from build123d import *

# Parameters (mm, degrees)
SKETCH1_W           = 130
SKETCH1_H           = 100
BOSS_EXTRUDE1_DEPTH = 51
SKETCH2_W           = 120
SKETCH2_H           = 90
CUT_EXTRUDE1_DEPTH  = 46
FILLET2_R           = 5
FILLET4_R           = 5
SKETCH6_W           = 5
SKETCH6_H           = 5
BOSS_EXTRUDE2_DEPTH = 20
BOSS_EXTRUDE3_DEPTH = 3


# Some blends are built 0.0001 mm under size
with BuildPart() as part:
    # Sketch1 → Boss-Extrude1 (new body)
    with BuildSketch(Plane(origin=(0, 0, 0), x_dir=(1, 0, 0), z_dir=(0, 1, 0))):
        Rectangle(SKETCH1_W, SKETCH1_H)
    extrude(amount=BOSS_EXTRUDE1_DEPTH)

    # Sketch2 → Cut-Extrude1 (cut)
    with BuildSketch(Plane(origin=(0, 51, 0), x_dir=(1, 0, 0), z_dir=(0, 1, 0))):
        Rectangle(SKETCH2_W, SKETCH2_H)
    extrude(amount=-CUT_EXTRUDE1_DEPTH, mode=Mode.SUBTRACT)

    # Fillet2
    fillet2_edges = [part.edges().sort_by_distance(p)[0] for p in [
        (-65, 51, 0),
        (0, 51, 50),
        (65, 51, 0),
        (0, 51, -50),
    ]]
    fillet(fillet2_edges, radius=FILLET2_R - 0.0001)  # a hair under: the kernel refuses the full size

    # Fillet4
    # the kernel refuses this fillet: 5 mm, written as the material it takes off along each edge
    with BuildSketch(Plane(origin=(60, 51, 45), x_dir=(0, 0, 1), z_dir=(-1, 0, 0))) as fillet4_piece_1:
        with BuildLine():
            CenterArc((0.0001, -4.9999), 4.9999, 0, 90)
            Line((5, -4.9999), (5, 0))
            Line((5, 0), (0.0001, 0))
        make_face()
    revolve(axis=Axis((60, 51, 45), (0, 1, 0)), revolution_arc=90, mode=Mode.SUBTRACT)
    with BuildSketch(Plane(origin=(-60, 51, 45), x_dir=(-1, 0, 0), z_dir=(0, 0, -1))) as fillet4_piece_2:
        with BuildLine():
            CenterArc((0.0001, -4.9999), 4.9999, 0, 90)
            Line((5, -4.9999), (5, 0))
            Line((5, 0), (0.0001, 0))
        make_face()
    revolve(axis=Axis((-60, 51, 45), (0, 1, 0)), revolution_arc=90, mode=Mode.SUBTRACT)
    with BuildSketch(Plane(origin=(60, 51, -45), x_dir=(1, 0, 0), z_dir=(0, 0, 1))) as fillet4_piece_3:
        with BuildLine():
            CenterArc((0.0001, -4.9999), 4.9999, 0, 90)
            Line((5, -4.9999), (5, 0))
            Line((5, 0), (0.0001, 0))
        make_face()
    revolve(axis=Axis((60, 51, -45), (0, 1, 0)), revolution_arc=90, mode=Mode.SUBTRACT)
    with BuildSketch(Plane(origin=(-60, 51, -45), x_dir=(0, 0, -1), z_dir=(1, 0, 0))) as fillet4_piece_4:
        with BuildLine():
            CenterArc((0.0001, -4.9999), 4.9999, 0, 90)
            Line((5, -4.9999), (5, 0))
            Line((5, 0), (0.0001, 0))
        make_face()
    revolve(axis=Axis((-60, 51, -45), (0, 1, 0)), revolution_arc=90, mode=Mode.SUBTRACT)
    with BuildSketch(Plane(origin=(-65, -12.5, -50), x_dir=(1, 0, 0), z_dir=(0, 1, 0)), Plane(origin=(-65, -12.5, 50), x_dir=(0, 0, -1), z_dir=(0, 1, 0))) as fillet4_piece_5:
        with BuildLine():
            CenterArc((FILLET4_R, -FILLET4_R), FILLET4_R, 90, 90)
            Line((0, -FILLET4_R), (0, 0))
            Line((0, 0), (FILLET4_R, 0))
        make_face()
    extrude(amount=63.5, mode=Mode.SUBTRACT)
    with BuildSketch(Plane(origin=(65, -12.5, -50), x_dir=(-1, 0, 0), z_dir=(0, 1, 0)), Plane(origin=(65, -12.5, 50), x_dir=(0, 0, -1), z_dir=(0, 1, 0))) as fillet4_piece_6:
        with BuildLine():
            CenterArc((FILLET4_R, FILLET4_R), FILLET4_R, 180, 90)
            Line((0, FILLET4_R), (0, 0))
            Line((0, 0), (FILLET4_R, 0))
        make_face()
    extrude(amount=63.5, mode=Mode.SUBTRACT)

    # Sketch6 → Boss-Extrude2 (add)
    with BuildSketch(Plane(origin=(0, 5, 0), x_dir=(1, 0, 0), z_dir=(0, 1, 0))):
        with Locations((-47.5, 32.5)):
            Rectangle(SKETCH6_W, SKETCH6_H)
        with Locations((-47.5, -31.53)):
            Rectangle(SKETCH6_W, SKETCH6_H)
        with Locations((1.77, 32.5)):
            Rectangle(SKETCH6_W, SKETCH6_H)
        with Locations((1.77, -31.53)):
            Rectangle(SKETCH6_W, SKETCH6_H)
    extrude(amount=BOSS_EXTRUDE2_DEPTH)

    # Sketch9 → Boss-Extrude3 (add)
    with BuildSketch(Plane(origin=(0, 5, 0), x_dir=(1, 0, 0), z_dir=(0, 1, 0))):
        Polygon((11.5, -14.03), (11.5, -19.03), (16.5, -19.03), (16.5, -18.03), (12.5, -18.03), (12.5, -14.03), align=None)
        Polygon((11.5, 27.97), (16.5, 27.97), (16.5, 26.97), (12.5, 26.97), (12.5, 22.97), (11.5, 22.97), align=None)
        Polygon((40, 27.97), (40, 22.97), (39, 22.97), (39, 26.97), (35, 26.97), (35, 27.97), align=None)
        Polygon((40, -19.03), (35, -19.03), (35, -18.03), (39, -18.03), (39, -14.03), (40, -14.03), align=None)
    extrude(amount=BOSS_EXTRUDE3_DEPTH)


solid = part.part
Here's how the part is built. I have some questions about the finished solid (model axes, mm). A direction names the side the tool comes from. Coordinates: 2 decimals unless noted, no trailing zeros. Order: outer loops, then holes, each group sorted by start corner. A loop starts at its lowest first (then second) coordinate and runs counter-clockwise, first axis right, second up. Notation, with made-up numbers: M 29,18 L 56,18 A24 ccw 56,49 Z; hole C 83,66 d9. An arc over 180 degrees is marked long. Answer as CSV lines item,"result".
Item 1: If I drill on line 1 (X direction, y = 8.5, z = 19); line 2 (Z direction, x = -52, y = 30); line 3 (X direction, y = 24.5, z = 32), over which ranges is the centre line in solid material (lowest first)?
Results found:
line 1,"-65 to -60, 60 to 65"
line 2,"-50 to -45, 45 to 50"
line 3,"-65 to -60, -50 to -45, -0.73 to 4.27, 60 to 65"
Item 2: We'd pull the mould along X, two halves only. Please class faces 3 (the face through (-48, 15, -30)), 4 (the face through (4.27, 15, 32)), 5 (the face through (-64, 23, 48)), 6 (the face through (1, 49, 49)): +X half, -X half, draft (parallel to the pull), parting line (faces both ways), or undercut.
Results found:
face 3,"undercut"
face 4,"undercut"
face 5,"-X half"
face 6,"draft"
Item 3: On a 3-axis mill with a long thin cutter (end or side, diameter ignored), from which of +Z, -Z, +X, -X, +Y, -Y can I reach the whole of each face in a straight line? I mean faces 1 (the face through (-0.73, 15, 32)), 2 (the face through (-1, 23, -50)). Say none if no direction works.
Results found:
face 1,"+Y"
face 2,"-Z, +X, -X, +Y, -Y"
Item 4: For pin 1 (3 mm diameter, centred on x = 17.5, z = -29.5, fed in from -Y); pin 2 (2.5 mm diameter, centred on x = 36.5, z = -26, fed in from +Y), each with a flat end and sliding along its axis, tell me the tip position at first contact or that it passes through.
Results found:
pin 1,"y = 0"
pin 2,"y = 8"
Item 5: Imagine slicing it at A-A on y = 20.5. Write out the boundary of the cut face in (x, z), plus the area to 3 significant figures.
Results found:
outline,"M -65,-45 A5 ccw -60,-50 L 60,-50 A5 ccw 65,-45 L 65,45 A5 ccw 60,50 L -60,50 A5 ccw -65,45 Z; M -50,-35 L -45,-35 L -45,-30 L -50,-30 Z; M -50,29.03 L -45,29.03 L -45,34.03 L -50,34.03 Z; M -0.73,-35 L 4.27,-35 L 4.27,-30 L -0.73,-30 Z; M -0.73,29.03 L 4.27,29.03 L 4.27,34.03 L -0.73,34.03 Z; hole M -60,-45 L 60,-45 L 60,45 L -60,45 Z"
area,"2,280 mm2"
Item 6: Imagine slicing it at C-C on y = 30. Write out the boundary of the cut face in (x, z).
Results found:
outline,"M -65,-45 A5 ccw -60,-50 L 60,-50 A5 ccw 65,-45 L 65,45 A5 ccw 60,50 L -60,50 A5 ccw -65,45 Z; hole M -60,-45 L 60,-45 L 60,45 L -60,45 Z"
